Input: dimensioned drawing with shaded views. Units: mm. Origin: part minimum x, y, z. A direction names the side the tool comes from. Coordinates: 2 decimals unless noted, no trailing zeros. Loops run counter-clockwise (first coordinate to the right, second up) from the corner with the lowest first, then second, coordinate; pieces in that order, holes last.
(1) Section A-A, the plane z = 5.75. Return loops of the section in (x, y) (1 decimal).
(2) Section B-B, the plane x = 21.5. Return loops of the section in (y, z) (1 decimal).
(3) Section C-C, the plane y = 98.5. Return loops of the section in (x, z) (1 decimal).
(4) Line query: L1, parallel to Y at x = 25.4, z = 23.2; L2, parallel to X at y = 81.5, z = 19.25 (1 decimal); L3, parallel to Z at x = 28, y = 204 (1 decimal). Output: solid intervals per line, ascending.
(5) Mould query, pull axis X, two halves, no side actions, for the marked faces 3, 4 and 5. Classes: released by +X, released by -X, zero draft, split by the parting line, or undercut.
(6) Section D-D, the plane x = 6. Return loops of the section in (y, z) (1 decimal).
(7) Set-up query: the marked faces 1 and 2. Return all of +Z, -Z, +X, -X, +Y, -Y with unobstructed straight access to the full face (end or side cutting, diameter ignored); none if empty.
(8) Contact query for flat-ended pins moving along their axis: P1, Ø1.5, axis at y = 168.5, z = 21.5, coming from the -X side; P2, Ø13.5, axis at x = 32.5, y = 100, coming from the -Z side (3 decimals). Output: stop coordinate, or through.
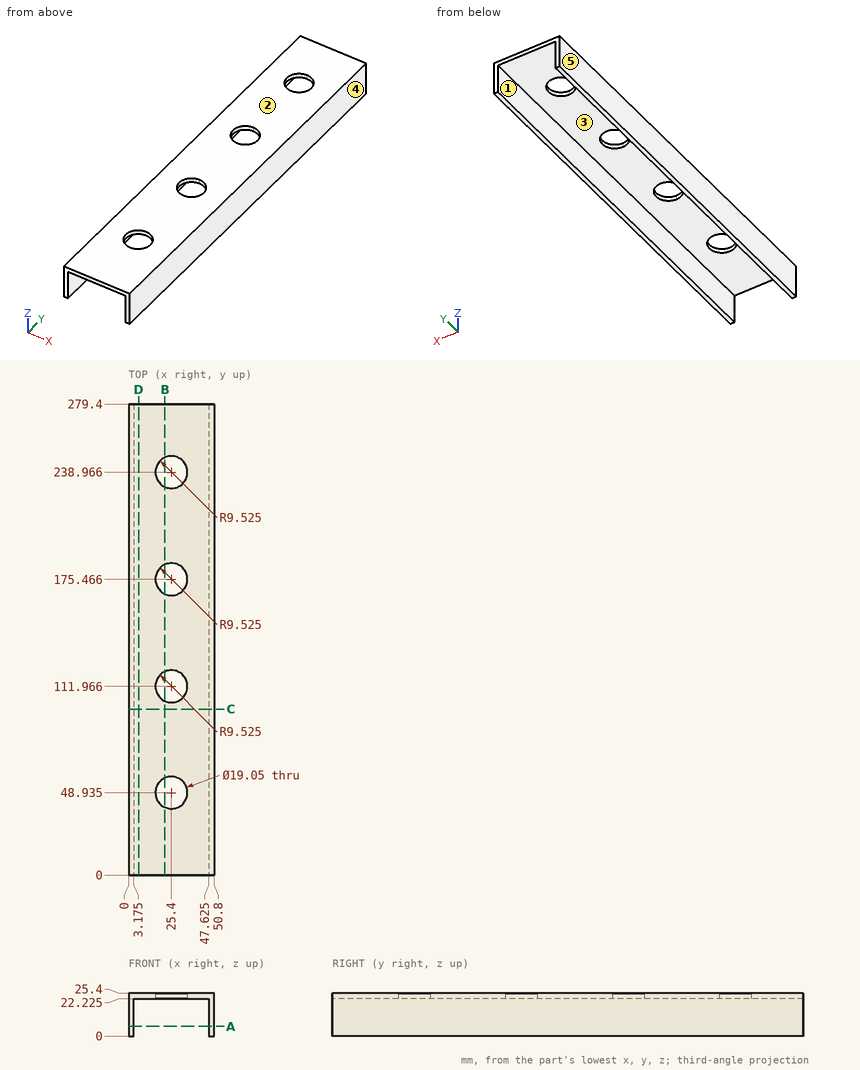
Report:
1. outline: (0, 0) - (3.2, 0) - (3.2, 279.4) - (0, 279.4) - close; (47.6, 0) - (50.8, 0) - (50.8, 279.4) - (47.6, 279.4) - close
2. outline: (0, 22.2) - (40.2, 22.2) - (40.2, 25.4) - (0, 25.4) - close; (57.6, 22.2) - (103.3, 22.2) - (103.3, 25.4) - (57.6, 25.4) - close; (120.7, 22.2) - (166.8, 22.2) - (166.8, 25.4) - (120.7, 25.4) - close; (184.2, 22.2) - (230.3, 22.2) - (230.3, 25.4) - (184.2, 25.4) - close; (247.7, 22.2) - (279.4, 22.2) - (279.4, 25.4) - (247.7, 25.4) - close
3. outline: (0, 0) - (3.2, 0) - (3.2, 22.2) - (47.6, 22.2) - (47.6, 0) - (50.8, 0) - (50.8, 25.4) - (0, 25.4) - close
4. L1: y = 0 to 39.41, 58.46 to 102.44, 121.49 to 165.94, 184.99 to 229.44, 248.49 to 279.4
4. L2: x = 0 to 3.2, 47.6 to 50.8
4. L3: z = 22.2 to 25.4
5. face 3: undercut
5. face 4: released by +X
5. face 5: released by -X
6. outline: (0, 22.2) - (279.4, 22.2) - (279.4, 25.4) - (0, 25.4) - close
7. face 1: -Z, +Y, -Y
7. face 2: +Z, +X, -X, +Y, -Y
8. P1: stops at x = 0
8. P2: stops at z = 22.225
